from build123d import *

# Parameters (mm, degrees)
F0_W         = 40
F0_H         = 70
F1_DEPTH     = 7
F2_R         = 5
F3_R         = 2
F4_DEPTH     = 3
F5_T1_DEPTH  = 60
F5_T3_DEPTH  = 30
F5_T6_ANGLE  = 90
F5_T8_ANGLE  = 90
F5_T10_ANGLE = 90
F5_T12_ANGLE = 90
F5_T14_ANGLE = 90
F5_T16_ANGLE = 90
F5_T18_ANGLE = 90
F5_T20_ANGLE = 90
F6_R         = 2.6271107644
F7_DEPTH     = 1


# Not quite as in the source:
# - a fillet or chamfer that OpenCascade refuses, or shapes differently, is made with other operations: its cross-section is extruded or revolved along the edge and cut away or added


with BuildPart() as f1:
    # F0 (on Top) → F1 (new body)
    with BuildSketch(Plane.XY):
        with Locations((20, 35)):
            Rectangle(F0_W, F0_H)
    extrude(amount=F1_DEPTH)

    # F2
    f2_edges = [f1.edges().sort_by_distance(p)[0] for p in [
        (40, 70, 3.5),
        (0, 70, 3.5),
        (40, 0, 3.5),
        (0, 0, 3.5),
    ]]
    fillet(f2_edges, radius=F2_R)

    # F3 (on face) → F4 (cut)
    with BuildSketch(Plane(origin=(0, 70, 0), x_dir=(-1, 0, 0), z_dir=(0, 1, 0))):
        with Locations((-29.8281734893, 3.5)):
            Circle(F3_R)
    extrude(amount=-F4_DEPTH, mode=Mode.SUBTRACT)

    # F5: fillet of radius 2 on 16 edges, made by hand

    # F5_s2 → F5_t1 (cut)
    with BuildSketch(Plane.XZ.offset(-65)):
        with BuildLine():
            ThreePointArc((0, 5), (0.5857864376, 6.4142135624), (2, 7))
            Line((2, 7), (0, 7))
            Line((0, 7), (0, 5))
        make_face()
        with BuildLine():
            ThreePointArc((0, 2), (0.5857864376, 0.5857864376), (2, 0))
            Line((2, 0), (0, 0))
            Line((0, 0), (0, 2))
        make_face()
        with BuildLine():
            ThreePointArc((38, 0), (39.4142135624, 0.5857864376), (40, 2))
            Line((40, 2), (40, 0))
            Line((40, 0), (38, 0))
        make_face()
        with BuildLine():
            ThreePointArc((38, 7), (39.4142135624, 6.4142135624), (40, 5))
            Line((40, 5), (40, 7))
            Line((40, 7), (38, 7))
        make_face()
    extrude(amount=F5_T1_DEPTH, mode=Mode.SUBTRACT)

    # F5_s4 → F5_t3 (cut)
    with BuildSketch(Plane.YZ.offset(5)):
        with BuildLine():
            ThreePointArc((68, 0), (69.4142135624, 0.5857864376), (70, 2))
            Line((70, 2), (70, 0))
            Line((70, 0), (68, 0))
        make_face()
        with BuildLine():
            ThreePointArc((2, 0), (0.5857864376, 0.5857864376), (0, 2))
            Line((0, 2), (0, 0))
            Line((0, 0), (2, 0))
        make_face()
        with BuildLine():
            ThreePointArc((68, 7), (69.4142135624, 6.4142135624), (70, 5))
            Line((70, 5), (70, 7))
            Line((70, 7), (68, 7))
        make_face()
        with BuildLine():
            ThreePointArc((2, 7), (0.5857864376, 6.4142135624), (0, 5))
            Line((0, 5), (0, 7))
            Line((0, 7), (2, 7))
        make_face()
    extrude(amount=F5_T3_DEPTH, mode=Mode.SUBTRACT)

    # F5_s5 → F5_t6 (revolve, cut)
    with BuildSketch(Plane.XZ.offset(-65)):
        with BuildLine():
            ThreePointArc((2, 0), (0.5857864376, 0.5857864376), (0, 2))
            Line((0, 2), (0, 0))
            Line((0, 0), (2, 0))
        make_face()
    revolve(axis=Axis((5, 65, 0), (0, 0, -1)), revolution_arc=F5_T6_ANGLE, mode=Mode.SUBTRACT)

    # F5_s7 → F5_t8 (revolve, cut)
    with BuildSketch(Plane.XZ.offset(-5)):
        with BuildLine():
            ThreePointArc((2, 0), (0.5857864376, 0.5857864376), (0, 2))
            Line((0, 2), (0, 0))
            Line((0, 0), (2, 0))
        make_face()
    revolve(axis=Axis((5, 5, 0), (0, 0, 1)), revolution_arc=F5_T8_ANGLE, mode=Mode.SUBTRACT)

    # F5_s9 → F5_t10 (revolve, cut)
    with BuildSketch(Plane.XZ.offset(-65)):
        with BuildLine():
            ThreePointArc((38, 0), (39.4142135624, 0.5857864376), (40, 2))
            Line((40, 2), (40, 0))
            Line((40, 0), (38, 0))
        make_face()
    revolve(axis=Axis((35, 65, 0), (0, 0, 1)), revolution_arc=F5_T10_ANGLE, mode=Mode.SUBTRACT)

    # F5_s11 → F5_t12 (revolve, cut)
    with BuildSketch(Plane.YZ.offset(35)):
        with BuildLine():
            ThreePointArc((2, 0), (0.5857864376, 0.5857864376), (0, 2))
            Line((0, 2), (0, 0))
            Line((0, 0), (2, 0))
        make_face()
    revolve(axis=Axis((35, 5, 0), (0, 0, 1)), revolution_arc=F5_T12_ANGLE, mode=Mode.SUBTRACT)

    # F5_s13 → F5_t14 (revolve, cut)
    with BuildSketch(Plane.XZ.offset(-65)):
        with BuildLine():
            ThreePointArc((0, 5), (0.5857864376, 6.4142135624), (2, 7))
            Line((2, 7), (0, 7))
            Line((0, 7), (0, 5))
        make_face()
    revolve(axis=Axis((5, 65, 7), (0, 0, -1)), revolution_arc=F5_T14_ANGLE, mode=Mode.SUBTRACT)

    # F5_s15 → F5_t16 (revolve, cut)
    with BuildSketch(Plane.XZ.offset(-5)):
        with BuildLine():
            ThreePointArc((0, 5), (0.5857864376, 6.4142135624), (2, 7))
            Line((2, 7), (0, 7))
            Line((0, 7), (0, 5))
        make_face()
    revolve(axis=Axis((5, 5, 7), (0, 0, 1)), revolution_arc=F5_T16_ANGLE, mode=Mode.SUBTRACT)

    # F5_s17 → F5_t18 (revolve, cut)
    with BuildSketch(Plane.XZ.offset(-65)):
        with BuildLine():
            ThreePointArc((38, 7), (39.4142135624, 6.4142135624), (40, 5))
            Line((40, 5), (40, 7))
            Line((40, 7), (38, 7))
        make_face()
    revolve(axis=Axis((35, 65, 7), (0, 0, 1)), revolution_arc=F5_T18_ANGLE, mode=Mode.SUBTRACT)

    # F5_s19 → F5_t20 (revolve, cut)
    with BuildSketch(Plane.YZ.offset(35)):
        with BuildLine():
            ThreePointArc((2, 7), (0.5857864376, 6.4142135624), (0, 5))
            Line((0, 5), (0, 7))
            Line((0, 7), (2, 7))
        make_face()
    revolve(axis=Axis((35, 5, 7), (0, 0, 1)), revolution_arc=F5_T20_ANGLE, mode=Mode.SUBTRACT)

    # F6 (on face) → F7 (cut)
    with BuildSketch(Plane.XY.offset(7)):
        with Locations((20, 6.6271107644)):
            Circle(F6_R)
    extrude(amount=-F7_DEPTH, mode=Mode.SUBTRACT)


solid = f1.part
Source: CAD feature listing. Evaluate the final solid. Frame: model axes, mm. A direction names the side the tool comes from. Give positions to 0.01 mm unless a question says otherwise; leave off trailing zeros. Write each loop counter-clockwise with the first axis right and the second up, starting at its lowest first coordinate (ties: lowest second). Pieces come first, ordered by that corner, then holes. Notation, with made-up numbers: (52, 2) - (83, 2) arc R26 cw to (83, 26) - close; hole circle Ø4 at (-32.5, -3.75). An arc over 180 degrees is marked (long way). Write item = value, one per line. Start each with the question number.
Q1. Pin query (flat end, axial travel): pin 1 Ø2.5 at (x, z) = (29.83, 3.5) entering from +Y; pin 2 Ø1.6 at (x, y) = (21, 5.5) entering from +Z. Return the tip coordinate at first contact, or that it passes through.
Q2. Cut plane A-A, the plane x = 20. Return loops of the section in (y, z), then the cut area to 3 significant figures.
Q3. Material intervals for probe 1 along Y at (x, z) = (19, 6.25); probe 2 along X at (y, z) = (69.35, 3.5); probe 3 along Y at (x, z) = (28.5, 1.5), sorted ascending.
Q4. Reachability of faces 5 (the flat face through (40, 35, 3)), 6 (the flat face through (20, 7, 6)) from +Z, -Z, +X, -X, +Y, -Y: full face, straight path, thin tool, end or side. Return the list, or none.
Q5. Cut plane B-B, the plane y = 8. Return loops of the section in (x, z).
Q6. Draft query along Z for faces 1 (the cylindrical face through (39, 68, 4)), 2 (the cylindrical face through (0.57, 35.42, 6.4)), 3 (the cylindrical face through (19.79, 0.6, 0.57)), 4 (the flat face through (30, 67, 4)). Return one class per face: +Z half, -Z half, draft (parallel to the pull), parting line (faces both ways), or undercut.
Computed values:
q1.pin_1 = 67
q1.pin_2 = 6
q2.outline = (0, 2) arc R2 ccw to (2, 0) - (68, 0) arc R2 ccw to (70, 2) - (70, 5) arc R2 ccw to (68, 7) - (9.25, 7) - (9.25, 6) - (4, 6) - (4, 7) - (2, 7) arc R2 ccw to (0, 5) - close
q2.area = 481 mm²
q3.probe_1 = 0.44 to 4.2, 9.06 to 69.56
q3.probe_2 = 2.53 to 27.83, 31.83 to 37.47
q3.probe_3 = 0.06 to 69.94
q4.face_5 = +Z, -Z, +X, +Y, -Y
q4.face_6 = +Z
q5.outline = (0, 2) arc R2 ccw to (2, 0) - (38, 0) arc R2 ccw to (40, 2) - (40, 5) arc R2 ccw to (38, 7) - (22.24, 7) - (22.24, 6) - (17.76, 6) - (17.76, 7) - (2, 7) arc R2 ccw to (0, 5) - close
q6.face_1 = draft
q6.face_2 = +Z half
q6.face_3 = -Z half
q6.face_4 = undercut
